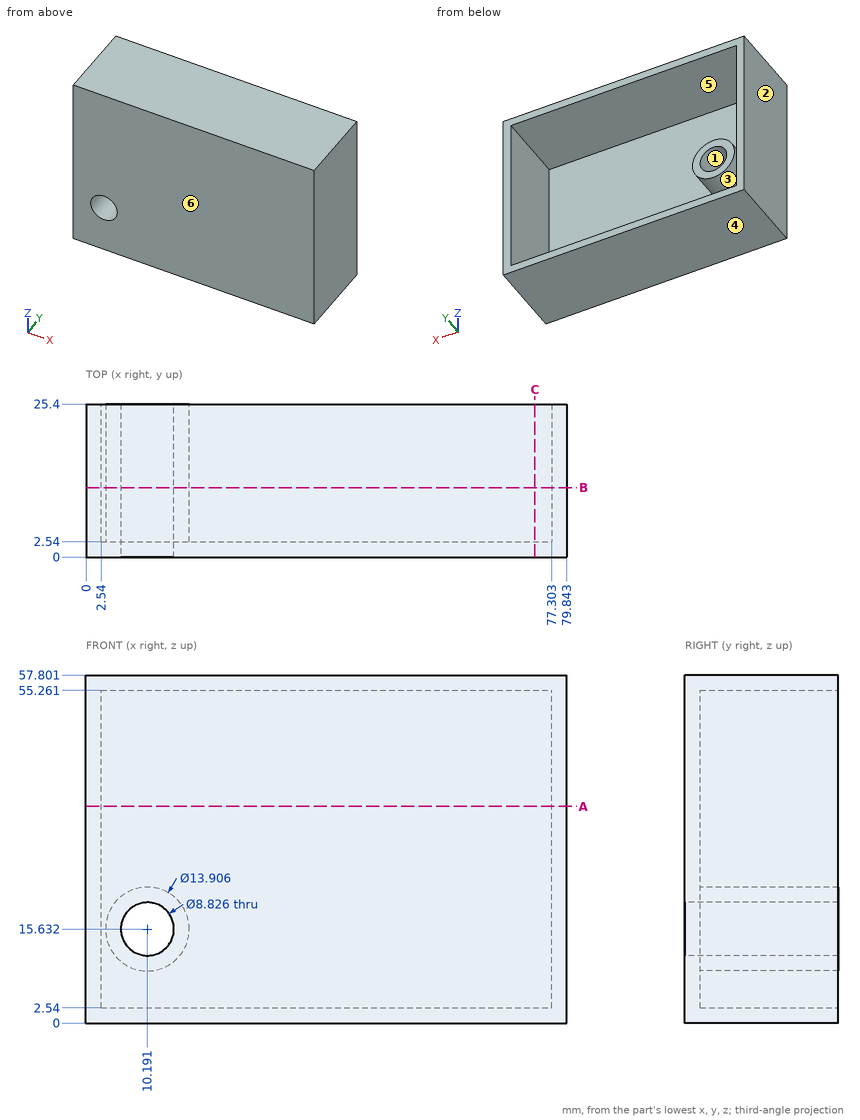
Study the drawing (mm; zero at the part's minimum x, y, z) and answer. A direction names the side the tool comes from. Give positions to 0.01 mm unless a question says otherwise; leave off trailing zeros. Write each loop counter-clockwise with the first axis right and the second up, starting at its lowest first coordinate (ties: lowest second). Pieces come first, ordered by that corner, then holes. Notation, with made-up numbers: (6, 75.25) -> (44, 75.25) arc R19 ccw to (44, 95.25) -> close; hole circle Ø2 at (66, 58.5). An arc over 180 degrees is marked (long way). Answer as a JSON object with one key per item and string values. Group by question number.
1) This flat-tipped pin is pushed along its axis until it touches: P1, Ø4, axis at x = 64.5, z = 25.5, coming from the +Y side. Where does it stop, or does it pass through?
2) The mould has two halves that part along Z. Classify the marked faces 1, 2, 3 and 4: +Z half, -Z half, draft (parallel to the pull), parting line (faces both ways), or undercut.
3) A tool of negligible diameter and unlimited length cuts with its end or side. For the marked faces 5 and 6, from which of +Z, -Z, +X, -X, +Y, -Y can it reach the whole face along a straight path? Write none if from no direction.
4) Find section B-B (y = 11.5). Write down the section's boundary in (x, z).
5) Find section A-A (z = 36). Write down the section's boundary in (x, y), and give its area (3 significant figures).
6) Consider L1, parallel to X at y = 12, z = 21 (1 decimal); L2, parallel to Z at x = 66, y = 19; L3, parallel to X at y = 17.25, z = 37. Determine where each line is inside the solid, lowest interval first. Write a range as from..to.
7) Find section C-C (x = 74.5). Write down the section's boundary in (y, z).
Values follow:
{
 "1": {"P1": "stops at y = 2.54"},
 "2": {"face 1": "undercut", "face 2": "draft", "face 3": "undercut", "face 4": "-Z half"},
 "3": {"face 5": "+Y", "face 6": "+Z, -Z, +X, -X, -Y"},
 "4": {"outline": "(0, 0) -> (79.84, 0) -> (79.84, 57.8) -> (0, 57.8) -> close; circle Ø13.91 at (10.19, 15.63); hole (2.54, 2.54) -> (77.3, 2.54) -> (77.3, 55.26) -> (2.54, 55.26) -> close; hole circle Ø8.83 at (10.19, 15.63)"},
 "5": {"outline": "(0, 0) -> (79.84, 0) -> (79.84, 25.4) -> (77.3, 25.4) -> (77.3, 2.54) -> (2.54, 2.54) -> (2.54, 25.4) -> (0, 25.4) -> close", "area": "319 mm2"},
 "6": {"L1": "x = 0..2.5, 5.8..14.6, 77.3..79.8", "L2": "z = 0..2.54, 55.26..57.8", "L3": "x = 0..2.54, 77.3..79.84"},
 "7": {"outline": "(0, 0) -> (25.4, 0) -> (25.4, 2.54) -> (2.54, 2.54) -> (2.54, 55.26) -> (25.4, 55.26) -> (25.4, 57.8) -> (0, 57.8) -> close"}
}
